Build history of the part. All positions in model axes, mm. Face numbers are marked on the shaded views. Round coordinates to 2 decimals unless told otherwise and drop trailing zeros. Order: outer loops, then holes, each group sorted by start corner. A loop starts at its lowest first (then second) coordinate and runs counter-clockwise, first axis right, second up. Notation, with made-up numbers: (-8.5, 14.5) -> (17.5, 14.5) arc R34 ccw to (17.5, 47.5) -> close; hole circle Ø6 at (64.25, 23.5). An arc over 180 degrees is marked (long way). Answer as a JSON object with one key per item and string values.
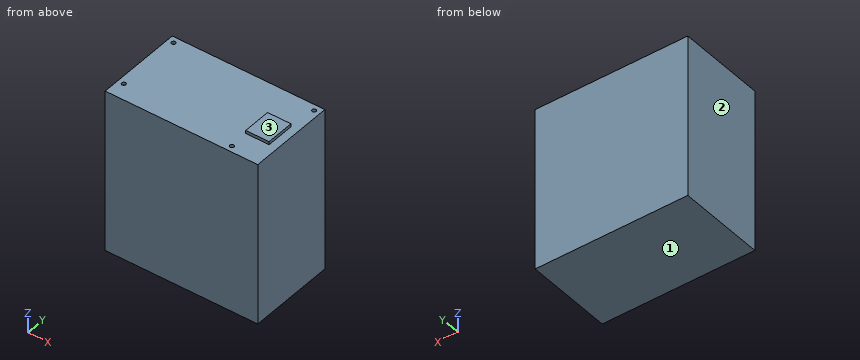
from build123d import *

# Parameters (mm, degrees)
SKETCH1_W           = 150
SKETCH1_H           = 160
BOSS_EXTRUDE1_DEPTH = 86
SKETCH6_W           = 23
SKETCH6_H           = 28
BOSS_EXTRUDE2_DEPTH = 3
SKETCH7_R           = 2
CUT_EXTRUDE1_DEPTH  = 3


with BuildPart() as part:
    # Sketch1 → Boss-Extrude1 (new body)
    with BuildSketch(Plane(origin=(0, 0, 0), x_dir=(1, 0, 0), z_dir=(0, 1, 0))):
        with Locations((75, 80)):
            Rectangle(SKETCH1_W, SKETCH1_H)
    extrude(amount=BOSS_EXTRUDE1_DEPTH)

    # Sketch6 → Boss-Extrude2 (add)
    with BuildSketch(Plane.XY):
        with Locations((130.5, 39)):
            Rectangle(SKETCH6_W, SKETCH6_H)
    extrude(amount=BOSS_EXTRUDE2_DEPTH)

    # Sketch7 → Cut-Extrude1 (cut)
    with BuildSketch(Plane.XY):
        with Locations((144, 80)):
            Circle(SKETCH7_R)
        with Locations(Location((6, 80, 0), (0, 0, 180))):
            Circle(SKETCH7_R)
        with Locations((6, 16)):
            Circle(SKETCH7_R)
        with Locations((120, 6)):
            Circle(SKETCH7_R)
    extrude(amount=-CUT_EXTRUDE1_DEPTH, mode=Mode.SUBTRACT)


solid = part.part
1) Cut at D-D, the plane y = 80. Give the cut face in (x, z).
Checked values:
{"outline": "(0, -160) -> (150, -160) -> (150, 0) -> (146, 0) -> (146, -3) -> (142, -3) -> (142, 0) -> (8, 0) -> (8, -3) -> (4, -3) -> (4, 0) -> (0, 0) -> close"}
2) Cut at B-B, the plane y = 42. Give the cut face in (x, z).
Checked values:
{"outline": "(0, -160) -> (150, -160) -> (150, 0) -> (142, 0) -> (142, 3) -> (119, 3) -> (119, 0) -> (0, 0) -> close"}
3) Probe L1, parallel to Y at x = 6, z = -1.9; L2, parallel to Y at x = 144, z = -2.2; L3, parallel to Y at x = 120, z = -1. List the from-to ranges inside material, lowest first. Write a range as from..to.
Checked values:
{"L1": "y = 0..14, 18..78, 82..86", "L2": "y = 0..78, 82..86", "L3": "y = 0..4, 8..86"}
4) Cut at A-A, the plane x = 144. Give the cut face in (y, z), plus the area to 3 significant figures.
Checked values:
{"outline": "(0, -160) -> (86, -160) -> (86, 0) -> (82, 0) -> (82, -3) -> (78, -3) -> (78, 0) -> (0, 0) -> close", "area": "13,700 mm²"}
5) Flat gauge pins, fed straight in: pin 1 Ø1.5 at (y, z) = (43, 1.5) entering from +X; pin 2 Ø1 at (x, y) = (103.5, 76.5) entering from +Z; pin 3 Ø0.9 at (y, z) = (44, 2) entering from -X. Where does each tip first touch, or does it go through?
Checked values:
{"pin 1": "stops at x = 142", "pin 2": "stops at z = 0", "pin 3": "stops at x = 119"}
6) Cut at C-C, the plane x = 6. Give the cut face in (y, z), plus the area to 3 significant figures.
Checked values:
{"outline": "(0, -160) -> (86, -160) -> (86, 0) -> (82, 0) -> (82, -3) -> (78, -3) -> (78, 0) -> (18, 0) -> (18, -3) -> (14, -3) -> (14, 0) -> (0, 0) -> close", "area": "13,700 mm²"}
7) Pull direction Z, two halves, no side cores. Call the marked faces 1, 2 and 3: pulls with the +Z half, pulls with the -Z half, needs draft (parallel to the pull), parting line crosses it, or undercut.
Checked values:
{"face 1": "pulls with the -Z half", "face 2": "needs draft", "face 3": "pulls with the +Z half"}
